```python
from build123d import *

# Parameters (mm, degrees)
F0_W     = 165.1
F0_H     = 31.75
F1_DEPTH = 21.3868
F2_W     = 38.1
F2_H     = 5.55625
F3_DEPTH = 31.75
F4_R     = 1.5875
F5_DEPTH = 21.3868


with BuildPart() as f1:
    # F0 (on Front) → F1 (new body)
    with BuildSketch(Plane.XZ):
        Rectangle(F0_W, F0_H)
    extrude(amount=F1_DEPTH)

    # F2 (on face) → F3 (cut, through all)
    with BuildSketch(Plane.XY.offset(15.875)):
        with Locations((63.5, -10.6934)):
            Rectangle(F2_W, F2_H)
    extrude(amount=-F3_DEPTH, mode=Mode.SUBTRACT)

    # F4 (on face) → F5 (cut, through all)
    with BuildSketch(Plane.XZ.offset(21.3868)):
        with Locations((60.325, 11.1125)):
            Circle(F4_R)
        with Locations((47.625, -11.1125)):
            Circle(F4_R)
    extrude(amount=-F5_DEPTH, mode=Mode.SUBTRACT)


solid = f1.part
```
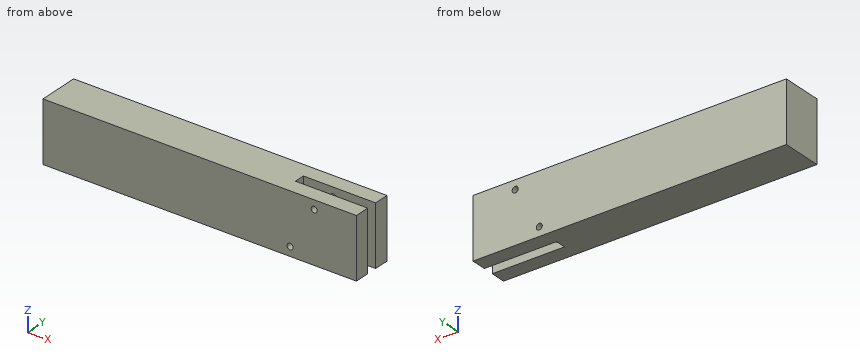
Work out the finished part from the listing and answer in its coordinate system (mm). Give positions to 0.01 mm unless a question says otherwise; leave off trailing zeros. Loops run counter-clockwise (first coordinate to the right, second up) from the corner with the lowest first, then second, coordinate; pieces in that order, holes last. Notation, with made-up numbers: (-37, 82) -> (-9, 82) arc R14 cw to (-9, 91) -> close; hole circle Ø7 at (36.5, 28.5). An arc over 180 degrees is marked (long way). One line per question, with ' | ' between items. Start each with the question number.
1) Straight lines are drawn through the part: L1, parallel to Y at x = 59, z = -10; L2, parallel to X at y = -8.5, z = -10. For each, find the intervals that lie inside material, in ascending order.
2) Section B-B, the plane z = -4.5 is taken. Determine the outline of the cut face in (x, y).
3) Section C-C, the plane y = -11.75 is taken. Determine the outline of the cut face in (x, z) (3 decimals), then the cut area to 3 significant figures.
4) Section A-A, the plane x = 63.5 is taken. Determine the outline of the cut face in (y, z) (3 decimals), then the cut area to 3 significant figures.
Resolved:
1) L1: -21.39 to -13.47, -7.92 to 0 | L2: -82.55 to 44.45
2) outline: (-82.55, -21.39) -> (82.55, -21.39) -> (82.55, -13.47) -> (44.45, -13.47) -> (44.45, -7.92) -> (82.55, -7.92) -> (82.55, 0) -> (-82.55, 0) -> close
3) outline: (-82.55, -15.875) -> (44.45, -15.875) -> (44.45, 15.875) -> (-82.55, 15.875) -> close | area: 4,030 mm2
4) outline: (-21.387, -15.875) -> (-13.472, -15.875) -> (-13.472, 15.875) -> (-21.387, 15.875) -> close; (-7.915, -15.875) -> (0, -15.875) -> (0, 15.875) -> (-7.915, 15.875) -> close | area: 503 mm2
